The model under review builds one solid part; all positions refer to its coordinate system, in mm. A direction names the side the tool comes from. Coordinates: 2 decimals unless noted, no trailing zeros. Write each loop counter-clockwise with the first axis right and the second up, starting at its lowest first coordinate (ties: lowest second). Pieces come first, ordered by that corner, then holes. Notation, with made-up numbers: M -36,46.25 L 4,46.25 A18 cw 4,73.25 Z; hole C 19,44 d11. An arc over 180 degrees is marked long. Answer as a JSON object with one key per item and string values.
Autodesk Fusion 360 part; units mm, degrees
sketch "Sketch1" plane through (0, 0, 0) normal (0, 0, 1) x (1, 0, 0)
  line L0 (-96.875, 55.375) -> (96.875, 55.375)
  line L1 (96.875, 55.375) -> (96.875, -55.375)
  line L2 (96.875, -55.375) -> (-96.875, -55.375)
  line L3 (-96.875, -55.375) -> (-96.875, 55.375)
  line L4 (-98.875, 57.375) -> (98.875, 57.375)
  line L5 (98.875, 57.375) -> (98.875, -57.375)
  line L6 (98.875, -57.375) -> (-98.875, -57.375)
  line L7 (-98.875, -57.375) -> (-98.875, 57.375)
  point P0 (0, 55.375)
  point P1 (-96.875, 0)
  point P2 (0, 57.375)
  point P3 (98.875, 0)
  dimension "d1" = 193.75
  dimension "d2" = 110.75
  dimension "d3" = 2
  dimension "d4" = 2
extrude "Extrude1" add sketch "Sketch1" along normal blind 14.8
sketch "Sketch2" plane through (0, 0, 0) normal (0, 0, -1) x (1, 0, 0)
  line L0 (-96.875, 55.375) -> (96.875, 55.375)
  line L1 (96.875, 55.375) -> (96.875, -55.375)
  line L2 (96.875, -55.375) -> (-96.875, -55.375)
  line L3 (-96.875, -55.375) -> (-96.875, 55.375)
  line L4 (98.875, 57.375) -> (-98.875, 57.375)
  line L5 (-98.875, 57.375) -> (-98.875, -57.375)
  line L6 (-98.875, -57.375) -> (98.875, -57.375)
  line L7 (98.875, -57.375) -> (98.875, 57.375)
  line L8 (-98.875, 57.375) -> (98.875, 57.375)
  line L9 (98.875, 57.375) -> (98.875, -57.375)
  line L10 (98.875, -57.375) -> (-98.875, -57.375)
  line L11 (-98.875, -57.375) -> (-98.875, 57.375)
  line L12 (-94.875, 53.375) -> (94.875, 53.375)
  line L13 (94.875, 53.375) -> (94.875, -53.375)
  line L14 (94.875, -53.375) -> (-94.875, -53.375)
  line L15 (-94.875, -53.375) -> (-94.875, 53.375)
  point P0 (0, 53.375)
  point P1 (94.875, 0)
  dimension "d15" = 2
  dimension "d16" = 2
extrude "Extrude2" add sketch "Sketch2" along normal blind 2 contours L0 L1 L2 L3 | L4 L5 L6 L7 L8 L9 L10 L11
fillet "Fillet1" radius 7.5 12 edges at (-94.875, -53.375, -1) (-94.875, 53.375, -1) (94.875, 53.375, -1) (94.875, -53.375, -1) (-98.875, 57.375, 6.4) (-98.875, -57.375, 6.4) (98.875, 57.375, 6.4) (98.875, -57.375, 6.4) (96.875, 55.375, 7.4) (96.875, -55.375, 7.4) (-96.875, -55.375, 7.4) (-96.875, 55.375, 7.4)
equation "d4 = d3"
equation "d5 = 2 mm + 4.8 mm + 8 mm"
equation "d16 = d15"
(1) For faces 4 (the face through (-1, 55.375, 7)), 5 (the face through (92.736, -51.12, -1.014)), 6 (the face through (-30, 55, -2)), list the 3-axis set-ups (+Z, -Z, +X, -X, +Y, -Y) from which the entire face can be reached by the end or side of a thin tool; tool diameter is ignored.
Results list:
{"face 4": "+Z", "face 5": "+Z, -Z", "face 6": "-Z, +X, -X, +Y, -Y"}
(2) Wall thickness on line 1 along Y through (x, z) = (-81, 2.5) (3 decimals); line 2 along Y through (x, z) = (16, -0.5) (3 decimals); line 3 along X through (y, z) = (22.5, -1.5) (3 decimals): over which ranges is each line inside the solid? List them lowest first. Write a range as from..to.
Results list:
{"line 1": "-57.375..-55.375, 55.375..57.375", "line 2": "-57.375..-53.375, 53.375..57.375", "line 3": "-98.875..-94.875, 94.875..98.875"}
(3) Add section B-B on y = -39.5. Give the boundary of the cut face in (x, z) (3 decimals), and give its area (3 significant figures).
Results list:
{"outline": "M -98.875,-2 L -94.875,-2 L -94.875,0 L -96.875,0 L -96.875,14.8 L -98.875,14.8 Z; M 94.875,-2 L 98.875,-2 L 98.875,14.8 L 96.875,14.8 L 96.875,0 L 94.875,0 Z", "area": "75.2 mm²"}
(4) Draft analysis for pull direction Y (two halves, no side actions). For faces 1 (the face through (1, -57.375, 6)), 2 (the face through (96.875, 1, 7)), 3 (the face through (-98.875, -1, 6)), state which applies: released by +Y, released by -Y, zero draft, split by the parting line, or undercut.
Results list:
{"face 1": "released by -Y", "face 2": "undercut", "face 3": "zero draft"}
(5) Add section A-A on x = 10.5. Give the boundary of the cut face in (y, z) (3 decimals).
Results list:
{"outline": "M -57.375,-2 L -53.375,-2 L -53.375,0 L -55.375,0 L -55.375,14.8 L -57.375,14.8 Z; M 53.375,-2 L 57.375,-2 L 57.375,14.8 L 55.375,14.8 L 55.375,0 L 53.375,0 Z"}
(6) Add section C-C on z = 5.25. Give the boundary of the cut face in (x, y) (3 decimals).
Results list:
{"outline": "M -98.875,-49.875 A7.5 ccw -91.375,-57.375 L 91.375,-57.375 A7.5 ccw 98.875,-49.875 L 98.875,49.875 A7.5 ccw 91.375,57.375 L -91.375,57.375 A7.5 ccw -98.875,49.875 Z; hole M -96.875,-47.875 A7.5 ccw -89.375,-55.375 L 89.375,-55.375 A7.5 ccw 96.875,-47.875 L 96.875,47.875 A7.5 ccw 89.375,55.375 L -89.375,55.375 A7.5 ccw -96.875,47.875 Z"}
